Source: three-view drawing plus pictorial views. Frame: mm from the lowest corner of the part. Coordinates: 2 decimals unless noted, no trailing zeros. Write each loop counter-clockwise with the first axis right and the second up, starting at its lowest first coordinate (ties: lowest second). Pieces come first, ordered by that corner, then holes. Notation, with made-up numbers: (79, 43.25) -> (138, 43.25) arc R35 cw to (138, 79.25) -> close; hole circle Ø10 at (84, 27.5). An arc over 180 degrees is marked (long way). One line per item, written item: value.
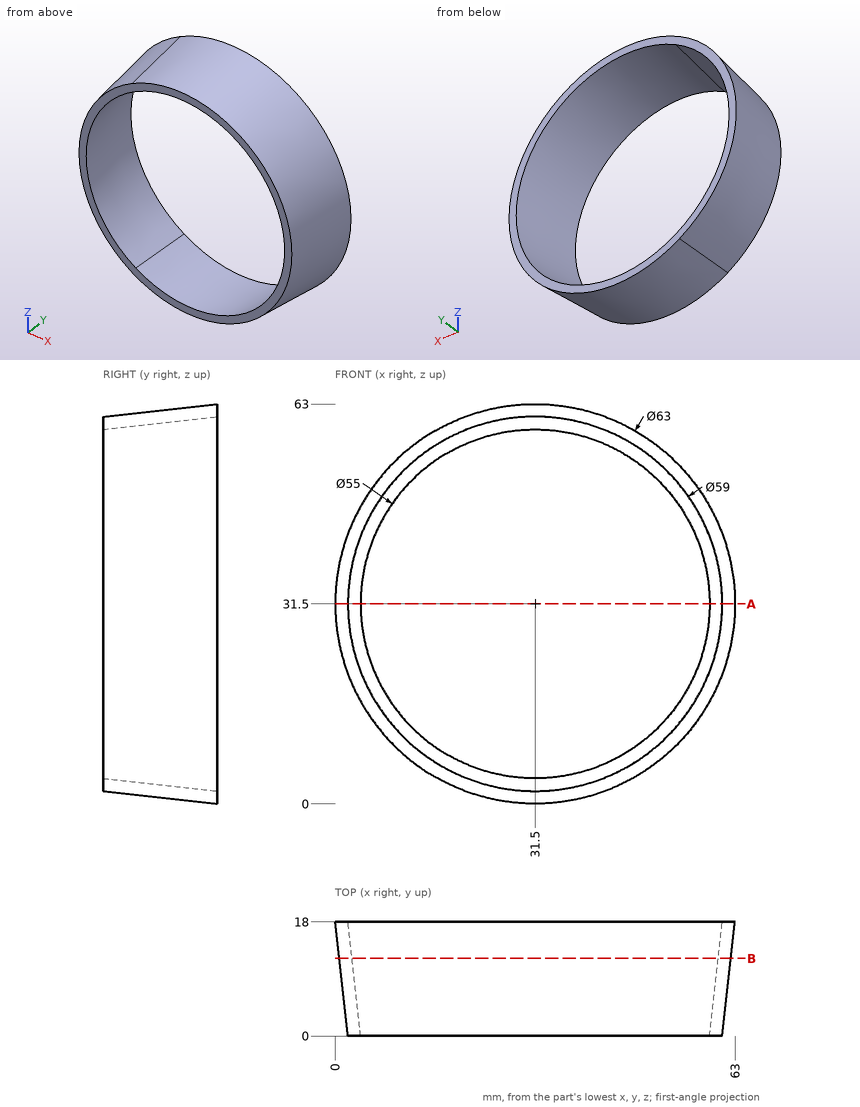
(1) Section A-A (z = 31.5). Return the cut outline in (x, y), then the cut area to 3 significant figures.
Responses:
outline: (0, 18) -> (2, 0) -> (4, 0) -> (2, 18) -> close; (59, 0) -> (61, 0) -> (63, 18) -> (61, 18) -> close
area: 72.0 mm2
(2) Line query: line 1 (Z direction, x = 26.5, y = 10); line 2 (Z direction, x = 47.5, y = 1.75); line 3 (X direction, y = 1.5, z = 16.5). Output: solid intervals per line, ascending. Write a range as [from, to].
Responses:
line 1: z = [1.3, 3.33], [59.67, 61.7]
line 2: z = [6.48, 8.9], [54.1, 56.52]
line 3: x = [5.9, 8.25], [54.75, 57.1]
(3) First-contact query: pin 1 (6 mm diameter, centred on y = 10.5, z = 51.5, fed in from -X); pin 2 (5 mm diameter, centred on x = 15, y = 5.5, fed in from -Z); pin 3 (5 mm diameter, centred on x = 22.5, y = 3, fed in from +Z). Flat tips, straight axial feed; report the tip coordinate or a pass-through.
Responses:
pin 1: stops at x = 5.94
pin 2: stops at z = 4.8
pin 3: stops at z = 60.68
(4) Section B-B (y = 12.25). Return the cut outline in (x, z), then the cut area to 3 significant figures.
Responses:
outline: circle Ø61.72 at (31.5, 31.5); hole (17.07, 6.51) arc R28.86 ccw (long way) to (17.07, 56.49) arc R28.86 ccw to start
area: 375 mm2
